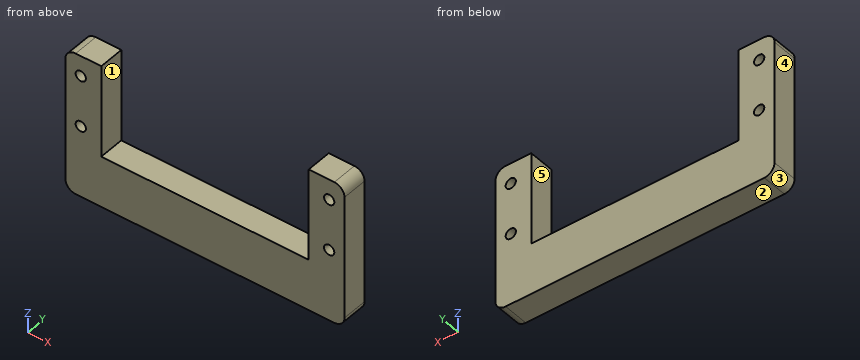
```python
from build123d import *

# Parameters (mm, degrees)
SKETCH1_R           = 1
BOSS_EXTRUDE2_DEPTH = 5
FILLET1_R           = 2


with BuildPart() as part:
    # Sketch1 → Boss-Extrude2 (new body)
    with BuildSketch(Plane(origin=(0, 0, 0), x_dir=(1, 0, 0), z_dir=(0, 1, 0))):
        with BuildLine():
            ThreePointArc((-25.25, -9), (-26.664213562, -8.414213562), (-27.25, -7))
            Line((-27.25, -7), (-27.25, 9))
            Line((-27.25, 9), (-20.25, 9))
            Line((-20.25, 9), (-20.25, -9))
            Line((-20.25, -9), (-25.25, -9))
        make_face()
        with Locations((-24.25, -5)):
            Circle(SKETCH1_R, mode=Mode.SUBTRACT)
        with Locations((-24.25, 5)):
            Circle(SKETCH1_R, mode=Mode.SUBTRACT)
        Polygon((-27.25, 9), (-20.25, 9), (20.25, 9), (27.25, 9), (27.25, 19), (-27.25, 19), align=None)
        with BuildLine():
            ThreePointArc((27.25, -7), (26.664213562, -8.414213562), (25.25, -9))
            Line((25.25, -9), (20.25, -9))
            Line((20.25, -9), (20.25, 9))
            Line((20.25, 9), (27.25, 9))
            Line((27.25, 9), (27.25, -7))
        make_face()
        with Locations((24.25, 5)):
            Circle(SKETCH1_R, mode=Mode.SUBTRACT)
        with Locations((24.25, -5)):
            Circle(SKETCH1_R, mode=Mode.SUBTRACT)
    extrude(amount=BOSS_EXTRUDE2_DEPTH)

    # Fillet1
    fillet1_edges = [part.edges().sort_by_distance(p)[0] for p in [
        (-27.25, 2.5, -19),
        (27.25, 2.5, -19),
    ]]
    fillet(fillet1_edges, radius=FILLET1_R)


solid = part.part
```
Here's how the part is built. I have some questions about the finished solid (model axes, mm). Face numbers are marked on the shaded views. A direction names the side the tool comes from. Coordinates: 2 decimals unless noted, no trailing zeros. Write each loop counter-clockwise with the first axis right and the second up, starting at its lowest first coordinate (ties: lowest second). Pieces come first, ordered by that corner, then holes. Notation, with made-up numbers: (-16, 70) -> (-5, 70) arc R14 cw to (-5, 95) -> close; hole circle Ø1 at (-33.5, 47). An arc over 180 degrees is marked (long way). Use a Markdown table: item, result. Add a question column.
(1) If we section it at D-D, the plane y = 3.7: Write out the boundary of the cut face in (x, z), and give its area (3 significant figures).
(2) If we section it at B-B, the plane z = -5: Write out the boundary of the cut face in (x, y).
(3) I'm going to push flat-ended pins straight in: P1, Ø1.6, axis at x = 24.25, z = -5, coming from the -Y side; P2, Ø3, axis at x = -18, y = 2, coming from the +Z side. Where does each tip first touch, or does it pass through?
(4) For the marked faces 4 and 5, which set-ups out of +Z, -Z, +X, -X, +Y, -Y let a thin tool reach every point of the face, with its end or its side?
(5) We'd pull the mould along X, two halves only. Please class the marked faces 1, 2 and 3: +X half, -X half, draft (parallel to the pull), parting line (faces both ways), or undercut.
(6) Please list where these lines run through material, in increasing order: line 1 (X direction, y = 1.9, z = -5); line 2 (Z direction, x = 24.25, y = 1.3); line 3 (X direction, y = 4.7, z = -6.75).
(7) If we section it at A-A, the plane x = -24.25: Write out the boundary of the cut face in (y, z).
(8) If we section it at C-C, the plane z = 0.5: Write out the boundary of the cut face in (x, y), and give its area (3 significant figures).
Outcome:
| question | item | result |
|---|---|---|
| 1 | outline | (-27.25, -17) arc R2 ccw to (-25.25, -19) -> (25.25, -19) arc R2 ccw to (27.25, -17) -> (27.25, 7) arc R2 ccw to (25.25, 9) -> (20.25, 9) -> (20.25, -9) -> (-20.25, -9) -> (-20.25, 9) -> (-25.25, 9) arc R2 ccw to (-27.25, 7) -> close; hole circle Ø2 at (-24.25, -5); hole circle Ø2 at (-24.25, 5); hole circle Ø2 at (24.25, -5); hole circle Ø2 at (24.25, 5) |
| 1 | area | 781 mm^2 |
| 2 | outline | (-27.25, 0) -> (-25.25, 0) -> (-25.25, 5) -> (-27.25, 5) -> close; (-23.25, 0) -> (-20.25, 0) -> (-20.25, 5) -> (-23.25, 5) -> close; (20.25, 0) -> (23.25, 0) -> (23.25, 5) -> (20.25, 5) -> close; (25.25, 0) -> (27.25, 0) -> (27.25, 5) -> (25.25, 5) -> close |
| 3 | P1 | passes through |
| 3 | P2 | stops at z = -9 |
| 4 | face 4 | +Z, -Z, -X, +Y, -Y |
| 4 | face 5 | +Z, +Y, -Y |
| 5 | face 1 | undercut |
| 5 | face 2 | draft |
| 5 | face 3 | -X half |
| 6 | line 1 | x = -27.25 to -25.25, -23.25 to -20.25, 20.25 to 23.25, 25.25 to 27.25 |
| 6 | line 2 | z = -19 to -6, -4 to 4, 6 to 9 |
| 6 | line 3 | x = -27.25 to -20.25, 20.25 to 27.25 |
| 7 | outline | (0, -19) -> (5, -19) -> (5, -6) -> (0, -6) -> close; (0, -4) -> (5, -4) -> (5, 4) -> (0, 4) -> close; (0, 6) -> (5, 6) -> (5, 9) -> (0, 9) -> close |
| 8 | outline | (-27.25, 0) -> (-20.25, 0) -> (-20.25, 5) -> (-27.25, 5) -> close; (20.25, 0) -> (27.25, 0) -> (27.25, 5) -> (20.25, 5) -> close |
| 8 | area | 70.0 mm^2 |
